Autodesk Inventor part; units mm, degrees
ref_plane "Work Plane1" through (-3, 0, -0.225) normal (-1, 0, 0) x (0, 0, 1)
ref_plane "YZ Plane" through (0, 0, 0) normal (1, 0, 0) x (0, 1, 0)
ref_plane "XZ Plane" through (0, 0, 0) normal (0, 1, 0) x (-1, 0, 0)
sketch "Sketch1" plane through (0, 0, 0) normal (0, 0, 1) x (1, 0, 0)
  line L0 (0, 4.5) -> (4.15, 4.5)
  line L1 (4.15, 4.5) -> (4.15, 0.5)
  line L2 (4.6, 0) -> (0, 0)
  line L3 (0, 0) -> (0, 4.5)
  line L4 (4.6, 0) -> (4.6, 0.5)
  line L5 (4.6, 0.5) -> (4.15, 0.5)
  dimension "d0" = 4.15
  dimension "d2" = 0.5
  dimension "d3" = 4.6
  dimension "d5" = 4.5
revolve "Revolution1" add sketch "Sketch1" angle 360 about axis through (0, 0, 0) along (0, 1, 0)
sketch "Sketch2" plane through (0, 4.5, 0) normal (0, 1, 0) x (1, 0, 0)
  line L0 (-2, 1.5) -> (2, 1.5)
  line L1 (2, 1.5) -> (2, -1.5)
  line L2 (2, -1.5) -> (-2, -1.5)
  line L3 (-2, -1.5) -> (-2, 1.5)
  line L4 (-2, 1.5) -> (2, -1.5) construction
  line L5 (2, 1.5) -> (-2, -1.5) construction
  point P0 (0, 0)
  dimension "d7" = 4
  dimension "d8" = 3
extrude "Extrusion1" cut sketch "Sketch2" against normal blind 0.5
sketch "Sketch3" plane through (0, 0, 0) normal (0, -1, 0) x (1, 0, 0)
  line L0 (-0.225, 0.225) -> (0.225, 0.225)
  line L1 (0.225, 0.225) -> (0.225, -0.225)
  line L2 (0.225, -0.225) -> (-0.225, -0.225)
  line L3 (-0.225, -0.225) -> (-0.225, 0.225)
  line L4 (-0.225, 0.225) -> (0.225, -0.225) construction
  line L5 (0.225, 0.225) -> (-0.225, -0.225) construction
  line L6 (2.775, 0.225) -> (3.225, 0.225)
  line L7 (3.225, 0.225) -> (3.225, -0.225)
  line L8 (3.225, -0.225) -> (2.775, -0.225)
  line L9 (2.775, -0.225) -> (2.775, 0.225)
  line L10 (2.775, 0.225) -> (3.225, -0.225) construction
  line L11 (3.225, 0.225) -> (2.775, -0.225) construction
  line L12 (-3.225, 0.225) -> (-2.775, 0.225)
  line L13 (-2.775, 0.225) -> (-2.775, -0.225)
  line L14 (-2.775, -0.225) -> (-3.225, -0.225)
  line L15 (-3.225, -0.225) -> (-3.225, 0.225)
  line L16 (-3.225, 0.225) -> (-2.775, -0.225) construction
  line L17 (-2.775, 0.225) -> (-3.225, -0.225) construction
  line L18 (-0.225, 0.225) -> (0.225, 0.225)
  line L19 (0.225, 0.225) -> (0.225, -0.225)
  line L20 (0.225, -0.225) -> (-0.225, -0.225)
  line L21 (-0.225, -0.225) -> (-0.225, 0.225)
  line L22 (-0.225, 0.225) -> (0.225, -0.225) construction
  line L23 (0.225, 0.225) -> (-0.225, -0.225) construction
  line L24 (-0.225, 3.225) -> (0.225, 3.225)
  line L25 (0.225, 3.225) -> (0.225, 2.775)
  line L26 (0.225, 2.775) -> (-0.225, 2.775)
  line L27 (-0.225, 2.775) -> (-0.225, 3.225)
  line L28 (-0.225, 3.225) -> (0.225, 2.775) construction
  line L29 (0.225, 3.225) -> (-0.225, 2.775) construction
  point P0 (0, 0)
  point P1 (3, 0)
  point P2 (-3, 0)
  point P3 (0, 0)
  point P4 (0, 3)
  point P5 (0, 0)
  point P6 (0, 0)
  dimension "d11" = 0.45
  dimension "d12" = 0.45
  dimension "d15" = 3
  dimension "d18" = 3
  dimension "d26" = 0.45
  dimension "d27" = 0.45
  dimension "d28" = 3
extrude "Extrusion2" add sketch "Sketch3" along normal blind 2 contours L6 L7 L8 L9 | L12 L13 L14 L15 | L24 L25 L26 L27
sketch "Sketch4" plane through (0, 0, 0) normal (0, -1, 0) x (1, 0, 0)
  line L0 (0, 0) -> (-4.5837, -4.5837)
  line L1 (0, 0) -> (-2.6627, 0)
  circle A0 centre (0, 0) radius 4.6
  line L2 (-3.0336, -3.4579) -> (-3.4579, -3.8822)
  line L3 (-3.4579, -3.8822) -> (-3.8822, -3.4579)
  line L4 (-3.8822, -3.4579) -> (-3.4579, -3.0336)
  point P0 (-3.67, -3.67)
  dimension "d29" = 45
  dimension "d30" = 0.6
  dimension "d31" = 0.6
extrude "Extrusion3" add sketch "Sketch4" against normal up to surface (0.5 mm away) contours A0 L2 L3 L0 | L0 L3 L4 A0
ref_plane "Work Plane1" through (-3, 0, -0.225) normal (-1, 0, 0) x (0, 0, 1)
sketch "Sketch6" plane through (-3, 0, -0.225) normal (-1, 0, 0) x (0, 0, 1)
  arc A0 (-0.475, -1.5) -> (0.225, -2.2) centre (0.225, -1.5) ccw
  line L0 (0, -2) -> (0.45, -2)
  line L1 (-0.475, -1.5) -> (0.225, -1.5)
  line L2 (0.225, -1.5) -> (0.225, -2.2)
  point P0 (0.225, 0)
  point P1 (0.225, -2)
  dimension "d36" = 0.5
  dimension "d37" = 0.7
revolve "Revolution2" add sketch "Sketch6" angle 360 about axis through (-3, -1.5, 0) along (0, -1, 0)
pattern_circular "Circular Pattern1" count 3 over 180 about axis through (0, 2.5, 0) along (0, 1, 0) of "Revolution2"
properties part number "PIR sensor RE200B"
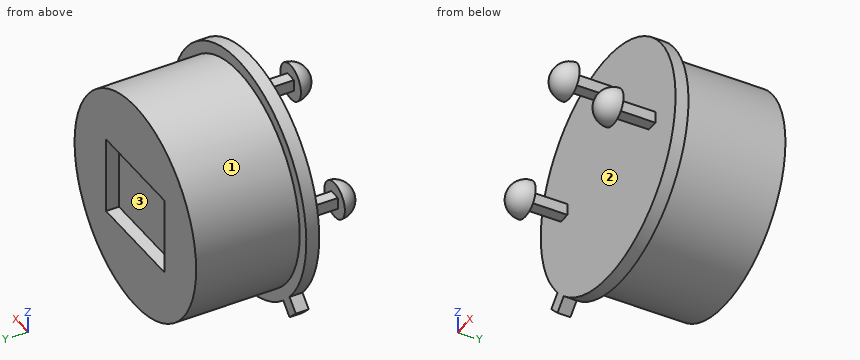
The model under review builds one solid part; all positions refer to its coordinate system, in mm. Face numbers are marked on the shaded views. Coordinates: 2 decimals unless noted, no trailing zeros. Loops run counter-clockwise (first coordinate to the right, second up) from the corner with the lowest first, then second, coordinate; pieces in that order, holes last. Notation, with made-up numbers: M 44.5,-18 L 92.5,-18 A19 ccw 92.5,8 Z; hole C 64,-34.5 d9. An arc over 180 degrees is marked long. Put each result on its own line as item: value. Start each with the question number.
Q1. Wall thickness on line 1 (Y direction, x = -3.75, z = 0.5); line 2 (Z direction, x = -0.5, y = 4.25); line 3 (Y direction, x = 1.75, z = -0.5): over which ranges is each line inside the solid? List them lowest first.
Q2. Clearance check with flat-ended pins moving along their axes: pin 1 (1 mm diameter, centred on x = -3.5, z = 3, fed in from -Y); pin 2 (0.5 mm diameter, centred on x = -3, y = -1, fed in from +Z) (3 decimals); pin 3 (1.5 mm diameter, centred on x = 0, z = 0, fed in from +Y). State where each tip first meets the part, or that it passes through.
Q3. Add section C-C (x = 2.5). Write out the cut boundary in (y, z).
Q4. Add section B-B (z = 0). Write out the cut boundary in (x, y) (3 decimals).
Q5. The part is to be moulded in two halves that separate along Z. For the marked faces 1, 2 and 3, say which applies: +Z half, -Z half, draft (parallel to the pull), parting line (faces both ways), or undercut.
Q6. Add section D-D (x = 0). Write out the cut boundary in (y, z) (3 decimals).
Q7. Add section A-A (y = -0.25). Write out the cut boundary in (x, z) (3 decimals), and give its area (4 significant figures).
Answers:
1. line 1: y = 0 to 4.5
1. line 2: z = -4.12 to -1.5, 1.5 to 4.12
1. line 3: y = 0 to 4
2. pin 1: stops at y = 0
2. pin 2: stops at z = 0.225
2. pin 3: stops at y = 4
3. outline: M -1.5,-0.49 L -1.5,0.49 A0.49 ccw Z; M 0,-3.86 L 0.5,-3.86 L 0.5,-3.31 L 4.5,-3.31 L 4.5,3.31 L 0.5,3.31 L 0.5,3.86 L 0,3.86 Z
4. outline: M -4.6,0 L -3.225,0 L -3.225,-1.5 L -3.7,-1.5 A0.7 ccw -2.3,-1.5 L -2.775,-1.5 L -2.775,0 L 2.775,0 L 2.775,-1.5 L 2.3,-1.5 A0.7 ccw 3.7,-1.5 L 3.225,-1.5 L 3.225,0 L 4.6,0 L 4.6,0.5 L 4.15,0.5 L 4.15,4.5 L 2,4.5 L 2,4 L -2,4 L -2,4.5 L -4.15,4.5 L -4.15,0.5 L -4.6,0.5 Z
5. face 1: parting line
5. face 2: draft
5. face 3: undercut
6. outline: M -1.5,2.3 L -1.5,2.775 L 0,2.775 L 0,-4.6 L 0.5,-4.6 L 0.5,-4.15 L 4.5,-4.15 L 4.5,-1.5 L 4,-1.5 L 4,1.5 L 4.5,1.5 L 4.5,4.15 L 0.5,4.15 L 0.5,4.6 L 0,4.6 L 0,3.225 L -1.5,3.225 L -1.5,3.7 A0.7 ccw Z
7. outline: M -3.225,-0.225 L -2.775,-0.225 L -2.775,0.225 L -3.225,0.225 Z; M -0.225,2.775 L 0.225,2.775 L 0.225,3.225 L -0.225,3.225 Z; M 2.775,-0.225 L 3.225,-0.225 L 3.225,0.225 L 2.775,0.225 Z
7. area: 0.6075 mm^2
